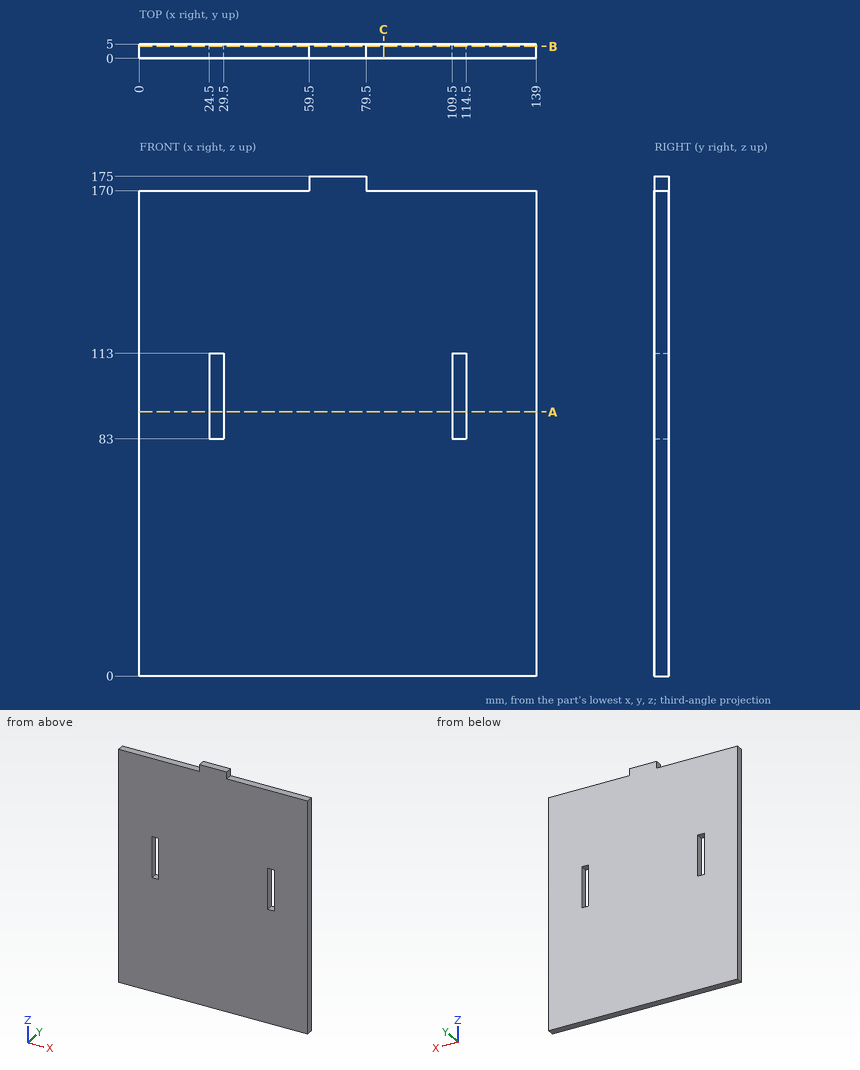
The figure shows three views and two pictorial views of one solid part (mm, origin at its lowest corner). Answer the questions. Coordinates: 2 decimals unless noted, no trailing zeros. Order: outer loops, then holes, each group sorted by start corner. A loop starts at its lowest first (then second) coordinate and runs counter-clockwise, first axis right, second up.
Q1. A cutting plane is placed at B-B, the plane y = 4.2. Write down the section's boundary in (x, z), and give its area (3 significant figures).
Q2. A cutting plane is placed at C-C, the plane x = 85.5. Write down the section's boundary in (y, z).
Q3. Given P1, Ø1.5, axis at x = 103, y = 1.5, coming from the +Z side; P2, Ø1.5, axis at x = 112.5, y = 2, coming from the -Z side; P3, Ø2.5, axis at y = 2, z = 173, coming from the +X side; P4, Ø2.5, axis at y = 2, z = 173, coming from the -X side, each flat-ended and moving along its own axis, determine where each tip first touches the part or whether it passes through.
Q4. Consider line 1 (X direction, y = 0.8, z = 91.5); line 2 (Z direction, x = 53.5, y = 4.7); line 3 (Z direction, x = 114, y = 2.9). Determine where each line is inside the solid, lowest interval first.
Q5. A cutting plane is placed at A-A, the plane z = 92.5. Write down the section's boundary in (x, y), and give its area (3 significant figures).
Answers follow:
1. outline: (0, 0) - (139, 0) - (139, 170) - (79.5, 170) - (79.5, 175) - (59.5, 175) - (59.5, 170) - (0, 170) - close; hole (24.5, 83) - (29.5, 83) - (29.5, 113) - (24.5, 113) - close; hole (109.5, 83) - (114.5, 83) - (114.5, 113) - (109.5, 113) - close
1. area: 23,400 mm2
2. outline: (0, 0) - (5, 0) - (5, 170) - (0, 170) - close
3. P1: stops at z = 170
3. P2: stops at z = 0
3. P3: stops at x = 79.5
3. P4: stops at x = 59.5
4. line 1: x = 0 to 24.5, 29.5 to 109.5, 114.5 to 139
4. line 2: z = 0 to 170
4. line 3: z = 0 to 83, 113 to 170
5. outline: (0, 0) - (24.5, 0) - (24.5, 5) - (0, 5) - close; (29.5, 0) - (109.5, 0) - (109.5, 5) - (29.5, 5) - close; (114.5, 0) - (139, 0) - (139, 5) - (114.5, 5) - close
5. area: 645 mm2
